from build123d import *
from build123d.topology import SkipClean

# Parameters (mm, degrees)
SKETCH1_R                               = 20
BOSS_EXTRUDE1_DEPTH                     = 20
BOSS_EXTRUDE2_START                     = -2
BOSS_EXTRUDE2_DEPTH                     = 2
CBORE_FOR_M8_HEX_HEAD_BOLT1_D           = 9
CBORE_FOR_M8_HEX_HEAD_BOLT1_CBORE_D     = 18.01
CBORE_FOR_M8_HEX_HEAD_BOLT1_CBORE_DEPTH = 6.68
M8X1_25_TAPPED_HOLE1_D                  = 6.8
M8X1_25_TAPPED_HOLE1_DEPTH              = 20
M8X1_25_TAPPED_HOLE1_TIP                = 2.042926105
CUT_EXTRUDE1_DEPTH                      = 58.035076926


with BuildPart() as part:
    # Sketch1 → Boss-Extrude1 (new body)
    with BuildSketch(Plane.XY):
        Polygon((-33, 42), (-33, -30), (33, -30), (33, 42), (18, 42), (11, 30), (-11, 30), (-18, 42), align=None)
        Circle(SKETCH1_R, mode=Mode.SUBTRACT)
    extrude(amount=BOSS_EXTRUDE1_DEPTH)

    # Sketch1_3 → Boss-Extrude2 (add)
    with SkipClean():  # the faces are left unmerged after this step: merging them gives an invalid solid
        with BuildSketch(Plane.XY.offset(BOSS_EXTRUDE2_START)):
            with BuildLine():
                ThreePointArc((-6e-09, 30), (-30, -1.1e-08), (1.5e-08, -30))
                Line((0, -30), (0, -20))
                ThreePointArc((0, -20), (-20, 0), (0, 20))
                Line((0, 20), (0, 30))
            make_face()
            with BuildLine():
                Line((0, -20), (0, -30))
                ThreePointArc((1.5e-08, -30), (21.213203441, -21.21320343), (30, 0))
                ThreePointArc((30, 0), (21.213203434, 21.213203438), (-6e-09, 30))
                Line((0, 30), (0, 20))
                ThreePointArc((0, 20), (14.142135624, 14.142135624), (20, 0))
                ThreePointArc((20, 0), (14.142135624, -14.142135624), (0, -20))
            make_face()
        extrude(amount=BOSS_EXTRUDE2_DEPTH)

    # CBORE for M8 Hex Head Bolt1 (through all)
    with Locations(Plane.XY.offset(20)):
        with Locations((-20, 15), (20, 15), (-20, -15), (20, -15)):
            CounterBoreHole(CBORE_FOR_M8_HEX_HEAD_BOLT1_D / 2, CBORE_FOR_M8_HEX_HEAD_BOLT1_CBORE_D / 2, CBORE_FOR_M8_HEX_HEAD_BOLT1_CBORE_DEPTH)

    # M8x1.25 Tapped Hole1
    with Locations(Plane.XY.offset(20)):
        with Locations((-25, 34), (25, 34), (25, 0), (-25, 0)):
            Hole(M8X1_25_TAPPED_HOLE1_D / 2, depth=M8X1_25_TAPPED_HOLE1_DEPTH)
            with Locations((0, 0, -(M8X1_25_TAPPED_HOLE1_DEPTH + M8X1_25_TAPPED_HOLE1_TIP / 2))):  # 118° drill point
                Cone(0, M8X1_25_TAPPED_HOLE1_D / 2, M8X1_25_TAPPED_HOLE1_TIP, mode=Mode.SUBTRACT)

    # Sketch7 → Cut-Extrude1 (cut, through all)
    with SkipClean():  # the faces are left unmerged after this step: merging them gives an invalid solid
        with BuildSketch(Plane(origin=(0, 0, 0), x_dir=(1, 0, 0), z_dir=(0, 1, 0))):
            with BuildLine():
                Line((-9, -20), (9, -20))
                Line((9, -20), (9, -10))
                ThreePointArc((9, -10), (7.242640687, -5.757359313), (3, -4))
                Line((3, -4), (-3, -4))
                ThreePointArc((-3, -4), (-7.242640687, -5.757359313), (-9, -10))
                Line((-9, -10), (-9, -20))
            make_face()
        extrude(amount=CUT_EXTRUDE1_DEPTH, mode=Mode.SUBTRACT)


solid = part.part
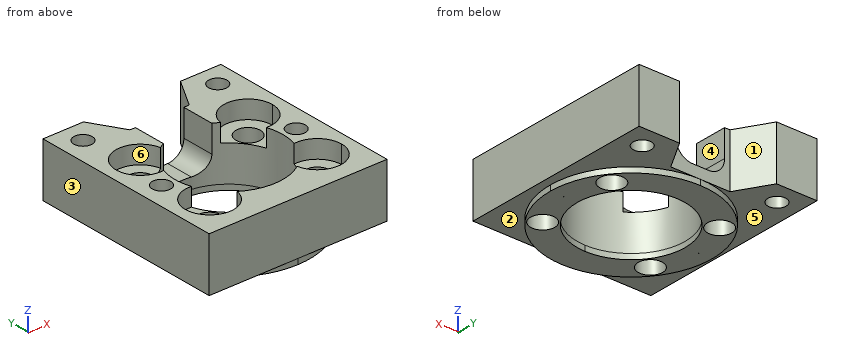
For this review, take the finished solid that the model builds, in its own axes (mm). Face numbers are marked on the shaded views. A direction names the side the tool comes from. Round coordinates to 2 decimals unless told otherwise and drop trailing zeros. Order: outer loops, then holes, each group sorted by start corner. A loop starts at its lowest first (then second) coordinate and runs counter-clockwise, first axis right, second up. Notation, with made-up numbers: M -17.5,21 L 36.5,21 A26 ccw 36.5,49 Z; hole C 42,58 d10. An arc over 180 degrees is marked long. Write each question's results on one line, items separated by ' | '. Start each with the question number.
1. Add section C-C (y = 29). State the section outline as (x, z) points, then the cut area to 3 significant figures.
2. To check wall thickness, follow L1, parallel to X at y = 0, z = 10; L2, parallel to X at y = 15, z = 18.5 (3 decimals); L3, parallel to X at y = 31, z = 18.75. State the ranges of each line that lie inside material, in increasing order. Write a range as [from, to].
3. Draft analysis for pull direction X (two halves, no side actions). For the marked faces 1, 2 and 3, state which applies: pulls with the +X half, pulls with the -X half, needs draft (parallel to the pull), parting line crosses it, or undercut.
4. Add section A-A (y = -18.5). State the section outline as (x, z) points, then the cut area to 3 significant figures.
5. Add section B-B (z = 12). State how many separate pieces and enclosed holes the cut face has, then the cut area to 3 significant figures.
6. Clearance check with flat-ended pins moving along their axes: pin 1 Ø4 at (x, y) = (-25, 34) entering from -Z; pin 2 Ø10 at (x, z) = (-5.5, 6) entering from +Y; pin 3 Ø4 at (x, y) = (-18.5, -18) entering from +Z; pin 4 Ø12 at (x, y) = (-2.5, 25) entering from +Z. State where each tip first meets the part, or that it passes through.
7. Tool access review of the marked faces 4, 5 and 6: name each direction out of +Z, -Z, +X, -X, +Y, -Y from which nothing blocks a thin tool from reaching the whole face with its end or side.
Output values:
1) outline: M -33,0 L -7.68,0 L -7.68,-2 L 7.68,-2 L 7.68,0 L 33,0 L 33,20 L 9,20 L 9,10 A6 cw 3,4 L -3,4 A6 cw -9,10 L -9,20 L -33,20 Z | area: 1,080 mm^2
2) L1: [-33, -28.4], [-21.6, -20], [20, 21.6], [28.4, 33] | L2: [-33, -29.005], [29.005, 33] | L3: [-33, -26.6], [-23.4, -11.58], [11.58, 23.4], [26.6, 33]
3) face 1: undercut | face 2: needs draft | face 3: pulls with the -X half
4) outline: M -33,0 L -23.62,0 L -23.62,-2 L -22.83,-2 L -22.83,13.32 L -28.3,13.32 L -28.3,20 L -33,20 Z; M -17.17,-2 L -7.6,-2 L -7.6,20 L -11.7,20 L -11.7,13.32 L -17.17,13.32 Z; M 7.6,-2 L 17.17,-2 L 17.17,13.32 L 11.7,13.32 L 11.7,20 L 7.6,20 Z; M 22.83,-2 L 23.62,-2 L 23.62,0 L 33,0 L 33,20 L 28.3,20 L 28.3,13.32 L 22.83,13.32 Z | area: 685 mm^2
5) separate pieces: 1 | enclosed holes: 8 | area: 2,560 mm^2
6) pin 1: through | pin 2: y = 30 | pin 3: z = 13.32 | pin 4: z = 7.6
7) face 4: +Z, +Y | face 5: -Z, -X | face 6: +Z
